Read the model definition and answer for the solid it produces. Units are mm, in the model's axes. Coordinates: 2 decimals unless noted, no trailing zeros. Loops run counter-clockwise (first coordinate to the right, second up) from the corner with the lowest first, then second, coordinate; pieces in that order, holes last. Notation, with made-up numbers: (-30.75, -27.75) -> (3.25, -27.75) arc R21 ccw to (3.25, -11.75) -> close; hole circle Ø6 at (-2, 80). An arc over 180 degrees is marked (long way). Answer as a JSON object with one key per item and string values. Group by question number.
1) Section C-C, the plane x = 44.45 is taken. Give the vertices of the cut face in (y, z), plus the area to 3 significant figures.
2) Section B-B, the plane x = 0 is taken. Give the vertices of the cut face in (y, z).
3) Section A-A, the plane y = -41.98 is taken. Give the vertices of the cut face in (x, z), plus the area to 3 significant figures.
4) Consider probe 1 along X at (y, z) = (-17, 0.7); probe 2 along X at (y, z) = (-2.5, 0.5); probe 3 along Y at (x, z) = (-31.75, 1.3). Determine where each line is inside the solid, lowest interval first. Write a range as [from, to].
5) Section D-D, the plane y = 10.5 is taken. Give the vertices of the cut face in (x, z).
6) Flat-ended cylindrical pins translate along their axes: P1, Ø1.5, axis at x = -10, z = 2, coming from the -Y side; P2, Ø4.5, axis at x = 31.75, y = -41.98, coming from the +Z side; P3, Ø2.5, axis at x = 44.45, y = 49.7, coming from the -Z side; P4, Ø0.9, axis at x = -10, z = 2, coming from the +Y side. Find the tip coordinate at first contact, or state that the pin passes through.
from build123d import *

# Parameters (mm, degrees)
SKETCH1_R           = 1.89865
BOSS_EXTRUDE3_DEPTH = 3.0988
SKETCH2_R           = 1.4732
CUT_EXTRUDE1_DEPTH  = 3.0988
CUT_EXTRUDE2_DEPTH  = 3.0988
SKETCH4_R           = 1.778
CUT_EXTRUDE3_DEPTH  = 3.0988


with BuildPart() as part:
    # Sketch1 → Boss-Extrude3 (new body)
    with BuildSketch(Plane.XY):
        with BuildLine():
            Line((-50.8, 55.175719298), (-50.8, -55.175719298))
            ThreePointArc((-50.8, -55.175719298), (0, -75), (50.8, -55.175719298))
            Line((50.8, -55.175719298), (50.8, 55.175719298))
            ThreePointArc((50.8, 55.175719298), (42.419210034, 61.851520758), (33.172661219, 67.264957799))
            ThreePointArc((33.172661219, 67.264957799), (0, 47.904876359), (-33.172661219, 67.264957799))
            ThreePointArc((-33.172661219, 67.264957799), (-42.419210034, 61.851520758), (-50.8, 55.175719298))
        make_face()
        with Locations((0, -66.675)):
            Circle(SKETCH1_R, mode=Mode.SUBTRACT)
        with Locations((-44.45, 49.6966108)):
            Circle(SKETCH1_R, mode=Mode.SUBTRACT)
        with Locations(Location((44.45, 49.6966108, 0), (0, 0, 180))):
            Circle(SKETCH1_R, mode=Mode.SUBTRACT)
    extrude(amount=BOSS_EXTRUDE3_DEPTH)

    # Sketch2 → Cut-Extrude1 (cut)
    with BuildSketch(Plane.XY.offset(3.0988)):
        with Locations((-31.75, -41.98)):
            Circle(SKETCH2_R)
        with Locations((31.75, -41.98)):
            Circle(SKETCH2_R)
        with Locations((-31.75, -9.1251)):
            Circle(SKETCH2_R)
        with Locations((31.75, -9.1251)):
            Circle(SKETCH2_R)
    extrude(amount=-CUT_EXTRUDE1_DEPTH, mode=Mode.SUBTRACT)

    # Sketch3 → Cut-Extrude2 (cut)
    with BuildSketch(Plane.XY.offset(3.0988)):
        with BuildLine():
            Line((8.827105782, 17.78), (2.54, 25.272680903))
            ThreePointArc((2.54, 25.272680903), (15.758317518, 19.920728626), (24.009298775, 8.289365013))
            Line((24.009298775, 8.289365013), (14.484298775, 8.647939367))
            Line((14.484298775, 8.647939367), (9.404298775, 5.715))
            Line((9.404298775, 5.715), (12.637105782, 17.78))
            Line((12.637105782, 17.78), (8.827105782, 17.78))
        make_face()
        with BuildLine():
            Line((18.868143133, -3.140634987), (24.826209076, 5.368365013))
            ThreePointArc((24.826209076, 5.368365013), (20.911260009, -14.418016674), (3.81, -25.112624315))
            Line((3.81, -25.112624315), (3.81, -14.877877919))
            Line((3.81, -14.877877919), (16.51, -14.877877919))
            Line((16.51, -14.877877919), (11.327081569, -9.797877919))
            Line((11.327081569, -9.797877919), (21.487081569, -4.935568543))
            Line((21.487081569, -4.935568543), (18.868143133, -3.140634987))
        make_face()
        with BuildLine():
            Line((-3.81, -14.877877919), (-3.81, -25.112624315))
            ThreePointArc((-3.81, -25.112624315), (-20.911260009, -14.418016674), (-24.826209076, 5.368365013))
            Line((-24.826209076, 5.368365013), (-18.868143133, -3.140634987))
            Line((-18.868143133, -3.140634987), (-21.487081569, -4.935568543))
            Line((-21.487081569, -4.935568543), (-11.327081569, -9.797877919))
            Line((-11.327081569, -9.797877919), (-16.51, -14.877877919))
            Line((-16.51, -14.877877919), (-3.81, -14.877877919))
        make_face()
        with BuildLine():
            Line((-14.484298775, 8.647939367), (-24.009298775, 8.289365013))
            ThreePointArc((-24.009298775, 8.289365013), (-15.758317518, 19.920728626), (-2.54, 25.272680903))
            Line((-2.54, 25.272680903), (-8.827105782, 17.78))
            Line((-8.827105782, 17.78), (-12.637105782, 17.78))
            Line((-12.637105782, 17.78), (-9.404298775, 5.715))
            Line((-9.404298775, 5.715), (-14.484298775, 8.647939367))
        make_face()
    extrude(amount=-CUT_EXTRUDE2_DEPTH, mode=Mode.SUBTRACT)

    # Sketch4 → Cut-Extrude3 (cut)
    with BuildSketch(Plane.XY.offset(3.0988)):
        with Locations((-34.29, 60.279957799)):
            Circle(SKETCH4_R)
        with Locations((34.29, 60.279957799)):
            Circle(SKETCH4_R)
        with Locations((34.29, 17.099957799)):
            Circle(SKETCH4_R)
        with Locations((-34.29, 17.099957799)):
            Circle(SKETCH4_R)
    extrude(amount=-CUT_EXTRUDE3_DEPTH, mode=Mode.SUBTRACT)


solid = part.part
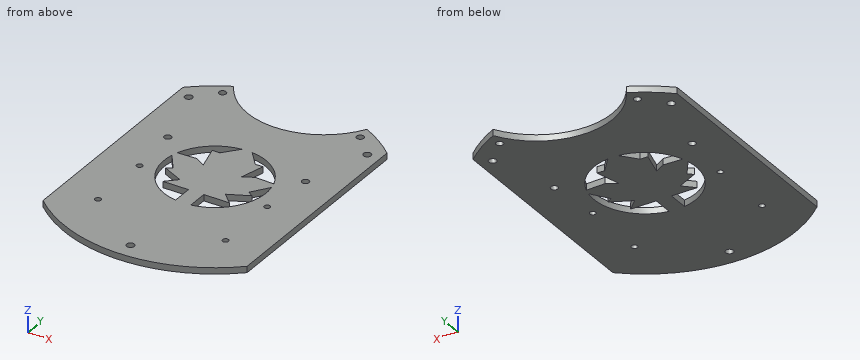
Determined:
{
 "1": {"outline": "(-60.41, 0) -> (47.8, 0) -> (47.8, 3.1) -> (-60.41, 3.1) -> close; (51.6, 0) -> (60.41, 0) -> (60.41, 3.1) -> (51.6, 3.1) -> close", "area": "363 mm²"},
 "2": {"outline": "(-75, 0) -> (-68.57, 0) -> (-68.57, 3.1) -> (-75, 3.1) -> close; (-64.78, 0) -> (47.9, 0) -> (47.9, 3.1) -> (-64.78, 3.1) -> close"},
 "3": {"outline": "(-50.8, 0) -> (-33.22, 0) -> (-33.22, 3.1) -> (-50.8, 3.1) -> close; (-30.28, 0) -> (30.28, 0) -> (30.28, 3.1) -> (-30.28, 3.1) -> close; (33.22, 0) -> (50.8, 0) -> (50.8, 3.1) -> (33.22, 3.1) -> close", "area": "297 mm²"},
 "4": {"probe 1": "[-50.8, -18.87], [-3.81, 3.81], [18.87, 50.8]", "probe 2": "[-50.8, -25.28], [-19.32, 19.32], [25.28, 50.8]", "probe 3": "[-67.95, -43.45], [-40.51, -10.6], [-7.65, 64.94]"},
 "5": {"outline": "(-50.8, 0) -> (-23.13, 0) -> (-23.13, 3.1) -> (-50.8, 3.1) -> close; (-10.69, 0) -> (10.69, 0) -> (10.69, 3.1) -> (-10.69, 3.1) -> close; (23.13, 0) -> (50.8, 0) -> (50.8, 3.1) -> (23.13, 3.1) -> close"},
 "6": {"P1": "y = -74.43", "P2": "z = 3.1", "P3": "through", "P4": "y = 49.37"}
}
